Check sheet for the modelled part. Datum: model origin and axes. Units: mm. Face numbers are marked on the shaded views. Round coordinates to 2 decimals unless told otherwise and drop trailing zeros. Write each loop counter-clockwise with the first axis right and the second up, starting at its lowest first coordinate (ties: lowest second). Pieces come first, ordered by that corner, then holes. Notation, with made-up numbers: M 52.25,59 L 108.25,59 A22 cw 108.25,77 Z; hole C 20,-37.75 d7. An arc over 180 degrees is marked long. One line per item, written item: value.
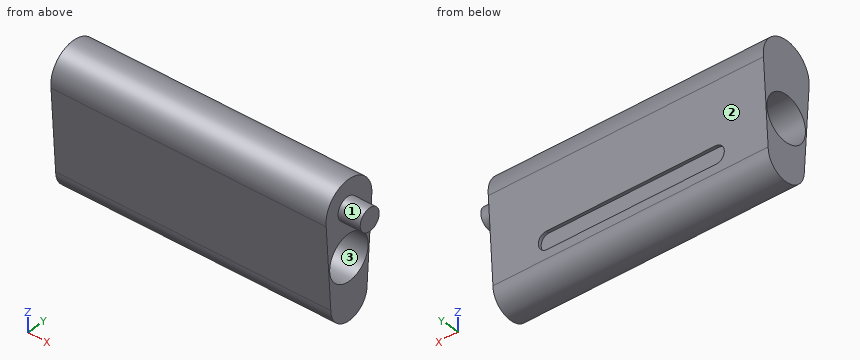
from build123d import *

# Parameters (mm, degrees)
BOSS_EXTRUDE1_DEPTH = 12.419249514
SKETCH3_R           = 1.015618984
CUT_EXTRUDE1_DEPTH  = 13.419249514
SKETCH4_R           = 0.5
BOSS_EXTRUDE4_DEPTH = 1
CUT_EXTRUDE4_DEPTH  = 0.15


with BuildPart() as part:
    # Sketch2 → Boss-Extrude1 (new body)
    with BuildSketch(Plane(origin=(0, 0, 0), x_dir=(0, 0, -1), z_dir=(1, 0, 0))):
        with BuildLine():
            Line((0.159499861, 1.199062904), (3.854352819, 0.954395011))
            ThreePointArc((3.854352819, 0.954395011), (4.80874783, 0), (3.854352819, -0.954395011))
            Line((3.854352819, -0.954395011), (0.159499861, -1.199062904))
            ThreePointArc((0.159499861, -1.199062904), (-1.209624757, 0), (0.159499861, 1.199062904))
        make_face()
    extrude(amount=BOSS_EXTRUDE1_DEPTH)

    # Sketch3 → Cut-Extrude1 (cut)
    with BuildSketch(Plane(origin=(12.419249514, 0, 0), x_dir=(0, 0, -1), z_dir=(1, 0, 0))):
        with Locations((2.120083087, 0)):
            Circle(SKETCH3_R)
    extrude(amount=-CUT_EXTRUDE1_DEPTH, mode=Mode.SUBTRACT)

    # Sketch4 → Boss-Extrude4 (add)
    with BuildSketch(Plane(origin=(12.419249514, -0.073237878, 0), x_dir=(0, 0, -1), z_dir=(1, 0, 0))):
        Circle(SKETCH4_R)
    extrude(amount=BOSS_EXTRUDE4_DEPTH)

    # Sketch7 → Cut-Extrude4 (cut)
    with BuildSketch(Plane(origin=(0, 1.20434383, -0.079749931), x_dir=(1, 0, 0), z_dir=(0, 0.9978147342638661, -0.06607386840446525))):
        with BuildLine():
            Line((2.310540733, 3.421811002), (9.955936015, 3.421811002))
            ThreePointArc((9.955936015, 3.421811002), (10.328984883, 3.048762133), (9.955936015, 2.675713265))
            Line((9.955936015, 2.675713265), (2.310540733, 2.675713265))
            ThreePointArc((2.310540733, 2.675713265), (1.937491864, 3.048762133), (2.310540733, 3.421811002))
        make_face()
    extrude(amount=-CUT_EXTRUDE4_DEPTH, mode=Mode.SUBTRACT)


solid = part.part
Q1. Sectioned sample at C-C on z = 0. Enter the section's corners in (x, y).
Completed:
outline: M 0,-1.21 L 12.42,-1.21 L 12.42,-0.57 L 13.42,-0.57 L 13.42,0.43 L 12.42,0.43 L 12.42,1.21 L 0,1.21 Z
Q2. Scan lines: line 1 (X direction, y = 0.25, z = -4); line 2 (Y direction, x = 7, z = -1.5); line 3 (Y direction, x = 10.5, z = -2.75). Record each from-to range of solid material in increasing order. Write a range as [from, to].
Completed:
line 1: [0, 12.42]
line 2: [-1.11, -0.8], [0.8, 1.11]
line 3: [-1.03, -0.8], [0.8, 1.03]
Q3. Draft check along Z on the marked faces 1, 2 and 3. Enter one of: pulls with the +Z half, pulls with the -Z half, needs draft (parallel to the pull), parting line crosses it, or undercut.
Completed:
face 1: parting line crosses it
face 2: pulls with the -Z half
face 3: undercut
Q4. Sectioned sample at D-D on x = 12.75. Enter the section's corners in (y, z), and give its area (3 significant figures).
Completed:
outline: C -0.07,0 d1
area: 0.785 mm^2
Q5. Sectioned sample at A-A on z = -2.25. Enter the section's corners in (x, y), and give its area (3 significant figures).
Completed:
outline: M 0,-1.06 L 12.42,-1.06 L 12.42,-1.01 L 0,-1.01 Z; M 0,1.01 L 12.42,1.01 L 12.42,1.06 L 0,1.06 Z
area: 1.33 mm^2
Q6. Sectioned sample at B-B on x = 7.75. Enter the section's corners in (y, z), and give its area (3 significant figures).
Completed:
outline: M -1.2,-0.16 L -0.95,-3.85 A0.95 ccw 0.95,-3.85 L 0.98,-3.49 L 0.83,-3.48 L 0.88,-2.74 L 1.03,-2.75 L 1.2,-0.16 A1.21 ccw long Z; hole C 0,-2.12 d2.03
area: 8.72 mm^2
